from build123d import *

# Parameters (mm, degrees)
SKETCH_1_W          = 190
SKETCH_1_H          = 167
EXTRUDE_1_DEPTH     = 1
CUT_EXTRUDE_1_DEPTH = 1
SKETCH_3_W          = 65
SKETCH_3_H          = 21
CUT_EXTRUDE_2_DEPTH = 1
SKETCH_4_R          = 1.6
CUT_EXTRUDE_3_DEPTH = 1
SKETCH_9_R          = 1.6
CUT_EXTRUDE_5_DEPTH = 10
FILLET_1_R          = 5
FILLET_2_R          = 2
SKETCH_10_R         = 1.6
CUT_EXTRUDE_6_DEPTH = 10
SKETCH_11_W         = 12
SKETCH_11_H         = 12
CUT_EXTRUDE_7_DEPTH = 10
FILLET_3_R          = 2
SKETCH_12_R         = 1.6
CUT_EXTRUDE_8_DEPTH = 10


with BuildPart() as part:
    # 草图1 → 凸台-拉伸1 (new body)
    with BuildSketch(Plane.XY):
        Rectangle(SKETCH_1_W, SKETCH_1_H)
    extrude(amount=EXTRUDE_1_DEPTH)

    # 草图2 → 切除-拉伸1 (cut)
    with BuildSketch(Plane(origin=(0, 0, 0), x_dir=(-1, 0, 0), z_dir=(0, 0, -1))):
        Polygon((100, -83.5), (119, -83.5), (119, 83.5), (55.252484864, 83.5), align=None)
    extrude(amount=-CUT_EXTRUDE_1_DEPTH, mode=Mode.SUBTRACT)

    # 草图3 → 切除-拉伸2 (cut)
    with BuildSketch(Plane(origin=(0, 0, 0), x_dir=(-1, 0, 0), z_dir=(0, 0, -1))):
        with Locations((62.5, -73)):
            Rectangle(SKETCH_3_W, SKETCH_3_H)
        Polygon((-88, 83.5), (55.252484864, 83.5), (70.123665044, 28), align=None)
    extrude(amount=-CUT_EXTRUDE_2_DEPTH, mode=Mode.SUBTRACT)

    # 草图4 → 切除-拉伸3 (cut)
    with BuildSketch(Plane(origin=(0, 0, 0), x_dir=(-1, 0, 0), z_dir=(0, 0, -1))):
        with Locations((-92, 4.5)):
            Circle(SKETCH_4_R)
        with Locations((-92, 24.5)):
            Circle(SKETCH_4_R)
    extrude(amount=-CUT_EXTRUDE_3_DEPTH, mode=Mode.SUBTRACT)

    # 草图9 → 切除-拉伸5 (cut)
    with BuildSketch(Plane(origin=(0, 0, 0), x_dir=(-1, 0, 0), z_dir=(0, 0, -1))):
        with Locations((-22.205756698, 57.227379318)):
            Circle(SKETCH_9_R)
        with Locations((-3.334428743, 50.603711057)):
            Circle(SKETCH_9_R)
    extrude(amount=-CUT_EXTRUDE_5_DEPTH, mode=Mode.SUBTRACT)

    # 圆角1
    fillet_1_edges = [part.edges().sort_by_distance(p)[0] for p in [
        (-30, -62.5, 0.5),
    ]]
    fillet(fillet_1_edges, radius=FILLET_1_R)

    # 圆角2
    fillet_2_edges = [part.edges().sort_by_distance(p)[0] for p in [
        (-94.373066959, -62.5, 0.5),
        (-70.123665044, 28, 0.5),
        (88, 83.5, 0.5),
        (-30, -83.5, 0.5),
        (95, -83.5, 0.5),
        (95, 83.5, 0.5),
    ]]
    fillet(fillet_2_edges, radius=FILLET_2_R)

    # 草图10 → 切除-拉伸6 (cut)
    with BuildSketch(Plane.XY.offset(1)):
        with Locations((45, -76.5)):
            Circle(SKETCH_10_R)
        with Locations((25, -76.5)):
            Circle(SKETCH_10_R)
    extrude(amount=-CUT_EXTRUDE_6_DEPTH, mode=Mode.SUBTRACT)

    # 草图11 → 切除-拉伸7 (cut)
    with BuildSketch(Plane(origin=(0, 0, 0), x_dir=(-1, 0, 0), z_dir=(0, 0, -1))):
        with Locations((-89, -77.5)):
            Rectangle(SKETCH_11_W, SKETCH_11_H)
    extrude(amount=-CUT_EXTRUDE_7_DEPTH, mode=Mode.SUBTRACT)

    # 圆角3
    fillet_3_edges = [part.edges().sort_by_distance(p)[0] for p in [
        (95, -71.5, 0.5),
        (83, -71.5, 0.5),
        (83, -83.5, 0.5),
    ]]
    fillet(fillet_3_edges, radius=FILLET_3_R)

    # 草图12 → 切除-拉伸8 (cut)
    with BuildSketch(Plane.XY.offset(1)):
        with Locations((-32.906682955, 33.75014876)):
            Circle(SKETCH_12_R)
        with Locations((-19.696753387, 38.386716542)):
            Circle(SKETCH_12_R)
        with Locations((37.860796874, 58.588904739)):
            Circle(SKETCH_12_R)
        with Locations((51.070726442, 63.225472522)):
            Circle(SKETCH_12_R)
    extrude(amount=-CUT_EXTRUDE_8_DEPTH, mode=Mode.SUBTRACT)


solid = part.part
Check sheet for the modelled part. Datum: model origin and axes. Units: mm. Round coordinates to 2 decimals unless told otherwise and drop trailing zeros. Loops run counter-clockwise (first coordinate to the right, second up) from the corner with the lowest first, then second, coordinate; pieces in that order, holes last. Notation, with made-up numbers: M -9,1 L 36,1 A17 ccw 36,19 Z; hole C 21,-11.5 d2. An arc over 180 degrees is marked long. One line per item, written item: value.
(1) Sectioned sample at B-B, the plane x = -44.5. Record the cut outline in (y, z), then the cut area to 3 significant figures.
Computed values:
outline: M -62.5,0 L 36.99,0 L 36.99,1 L -62.5,1 Z
area: 99.5 mm^2
(2) Sectioned sample at A-A, the plane z = 0.5. Count the separate pieces of the cut face and the enclosed holes in it, then the cut area to 3 significant figures.
Computed values:
separate pieces: 1
enclosed holes: 10
area: 23,200 mm^2
(3) Depth check by flat-ended pin: pin 1 Ø0.5 at (x, z) = (88, 0.5) entering from -Y; pin 2 Ø0.5 at (y, z) = (-73, 0.5) entering from -X. Enter the tip coordinate at first touch or a pass-through.
Computed values:
pin 1: stops at y = -71.5
pin 2: stops at x = -30
(4) Sectioned sample at C-C, the plane y = -28. Record the cut outline in (x, z), then the cut area to 3 significant figures.
Computed values:
outline: M -85.13,0 L 95,0 L 95,1 L -85.13,1 Z
area: 180 mm^2
(5) Thickness scan on line 1 (X direction, y = -76.5, z = 0.5); line 2 (Y direction, x = 25, z = 0.75); line 3 (Y direction, x = 45, z = 0.3). Record the ranges inside material, lowest first.
Computed values:
line 1: x = -30 to 23.4, 26.6 to 43.4, 46.6 to 83
line 2: y = -83.5 to -78.1, -74.9 to 61.39
line 3: y = -83.5 to -78.1, -74.9 to 68.41
